from build123d import *

# Parameters (mm, degrees)
F0_W     = 10
F0_H     = 10
F0_R     = 1.25
F1_DEPTH = 10


with BuildPart() as f1:
    # F0 (on Front) → F1 (new body)
    with BuildSketch(Plane.XZ):
        Rectangle(F0_W, F0_H)
        with Locations((-3.125, -3.125)):
            Circle(F0_R, mode=Mode.SUBTRACT)
        with Locations((0, -3.125)):
            Circle(F0_R, mode=Mode.SUBTRACT)
        with Locations((3.125, -3.125)):
            Circle(F0_R, mode=Mode.SUBTRACT)
        with Locations((-3.125, 0)):
            Circle(F0_R, mode=Mode.SUBTRACT)
        with Locations((-3.125, 3.125)):
            Circle(F0_R, mode=Mode.SUBTRACT)
        Circle(F0_R, mode=Mode.SUBTRACT)
        with Locations((3.125, 0)):
            Circle(F0_R, mode=Mode.SUBTRACT)
        with Locations((0, 3.125)):
            Circle(F0_R, mode=Mode.SUBTRACT)
        with Locations((3.125, 3.125)):
            Circle(F0_R, mode=Mode.SUBTRACT)
    extrude(amount=F1_DEPTH)


solid = f1.part
For this review, take the finished solid that the model builds, in its own axes (mm). Round coordinates to 2 decimals unless told otherwise and drop trailing zeros. Loops run counter-clockwise (first coordinate to the right, second up) from the corner with the lowest first, then second, coordinate; pieces in that order, holes last. Notation, with made-up numbers: (13, 85) - (56, 85) arc R12 ccw to (56, 97) - close; hole circle Ø6 at (49.5, 9.5). An arc over 180 degrees is marked (long way). One line per item, written item: value. Start each with the question number.
Item 1: Take a section at A-A (z = 0). Give the boundary of the cut face in (x, y) (3 decimals), plus the area to 3 significant figures.
Item 2: Take a section at B-B (x = 0). Give the boundary of the cut face in (y, z) (3 decimals), plus the area to 3 significant figures.
Item 3: For L1, parallel to X at y = -8.25, z = -0.25; L2, parallel to X at y = -6.5, z = 0.75 (3 decimals); L3, parallel to Z at x = 0, y = -4.75 (3 decimals), list the stretches that pass through material, from the lowest coordinate up.
Item 4: The part is to be moulded in two halves that separate along Z. For faces 1 (the flat face through (0, -5, 5)), 2 (the flat face through (5, -5, 0)), 3 (the cylindrical face through (-0.27, -4.93, -1.22)), say which applies: +Z half, -Z half, draft (parallel to the pull), parting line (faces both ways), or undercut.
Answer below:
1. outline: (-5, -10) - (-4.375, -10) - (-4.375, 0) - (-5, 0) - close; (-1.875, -10) - (-1.25, -10) - (-1.25, 0) - (-1.875, 0) - close; (1.25, -10) - (1.875, -10) - (1.875, 0) - (1.25, 0) - close; (4.375, -10) - (5, -10) - (5, 0) - (4.375, 0) - close
1. area: 25.0 mm2
2. outline: (-10, -5) - (0, -5) - (0, -4.375) - (-10, -4.375) - close; (-10, -1.875) - (0, -1.875) - (0, -1.25) - (-10, -1.25) - close; (-10, 1.25) - (0, 1.25) - (0, 1.875) - (-10, 1.875) - close; (-10, 4.375) - (0, 4.375) - (0, 5) - (-10, 5) - close
2. area: 25.0 mm2
3. L1: x = -5 to -4.35, -1.9 to -1.22, 1.22 to 1.9, 4.35 to 5
3. L2: x = -5 to -4.125, -2.125 to -1, 1 to 2.125, 4.125 to 5
3. L3: z = -5 to -4.375, -1.875 to -1.25, 1.25 to 1.875, 4.375 to 5
4. face 1: +Z half
4. face 2: draft
4. face 3: undercut
